The model under review builds one solid part; all positions refer to its coordinate system, in mm. A direction names the side the tool comes from. Give positions to 0.01 mm unless a question says otherwise; leave off trailing zeros. Write each loop counter-clockwise with the first axis right and the second up, starting at its lowest first coordinate (ties: lowest second). Pieces come first, ordered by that corner, then holes. Notation, with made-up numbers: (62, -35) -> (71, -35) arc R16 ccw to (71, -18) -> close; hole circle Ø7 at (56, 57.5). An arc over 180 degrees is marked (long way). Use CSV: the item, a comma, the result in double quotes.
```python
from build123d import *

# Parameters (mm, degrees)
BOSS_EXTRUDE1_DEPTH     = 9.525
SKETCH12_R              = 2.75
CUT_EXTRUDE2_DEPTH      = 278.704385318
CUT_EXTRUDE3_DEPTH      = 291.894698516
CUT_EXTRUDE3_DEPTH_BACK = 291.894698516
SKETCH13_R              = 2.75
SKETCH14_R              = 5
CUT_EXTRUDE4_DEPTH      = 291.894698516


with BuildPart() as part:
    # Sketch1 → Boss-Extrude1 (new, symmetric)
    with BuildSketch(Plane.XY):
        with BuildLine():
            Line((50, 0), (50, 243))
            ThreePointArc((50, 243), (41.213203436, 264.213203436), (20, 273))
            Line((20, 273), (-20, 273))
            ThreePointArc((-20, 273), (-41.213203436, 264.213203436), (-50, 243))
            Line((-50, 243), (-50, 0))
            Line((-50, 0), (-46.825, 0))
            Line((-46.825, 0), (-46.825, 243))
            ThreePointArc((-46.825, 243), (-38.968139405, 261.968139405), (-20, 269.825))
            Line((-20, 269.825), (20, 269.825))
            ThreePointArc((20, 269.825), (38.968139405, 261.968139405), (46.825, 243))
            Line((46.825, 243), (46.825, 0))
            Line((46.825, 0), (50, 0))
        make_face()
    extrude(amount=BOSS_EXTRUDE1_DEPTH, both=True)

    # Sketch12 → Cut-Extrude2 (cut, through all)
    with BuildSketch(Plane(origin=(0, 273, 0), x_dir=(1, 0, 0), z_dir=(0, 1, 0))):
        with Locations(Location((0, 0, 0), (0, 0, 270))):
            Circle(SKETCH12_R)
        with Locations(Location((-15, 0, 0), (0, 0, 270))):
            Circle(SKETCH12_R)
        with Locations(Location((15, 0, 0), (0, 0, 270))):
            Circle(SKETCH12_R)
    extrude(amount=-CUT_EXTRUDE2_DEPTH, mode=Mode.SUBTRACT)

    # Sketch13 → Cut-Extrude3 (cut, two sides: drawn at the far end of the back side and taken through both)
    with BuildSketch(Plane(origin=(50, 0, 0), x_dir=(0, 0, -1), z_dir=(1, 0, 0)).offset(-CUT_EXTRUDE3_DEPTH_BACK)):
        with Locations((0, 220)):
            Circle(SKETCH13_R)
        with Locations((0, 125)):
            Circle(SKETCH13_R)
        with Locations((0, 55)):
            Circle(SKETCH13_R)
    extrude(amount=CUT_EXTRUDE3_DEPTH + CUT_EXTRUDE3_DEPTH_BACK, mode=Mode.SUBTRACT)

    # Sketch14 → Cut-Extrude4 (cut, through all)
    with BuildSketch(Plane(origin=(50, 0, 0), x_dir=(0, 0, -1), z_dir=(1, 0, 0))):
        with Locations((0, 234.175)):
            Circle(SKETCH14_R)
    extrude(amount=-CUT_EXTRUDE4_DEPTH, mode=Mode.SUBTRACT)


solid = part.part
```
Q1. Consider section B-B (x = -15). Write out the cut boundary in (y, z) (3 decimals).
Derived:
outline,"(269.825, -9.525) -> (273, -9.525) -> (273, -2.75) -> (269.825, -2.75) -> close; (269.825, 2.75) -> (273, 2.75) -> (273, 9.525) -> (269.825, 9.525) -> close"
Q2. Insertion check: pin 1 (6.5 mm diameter, centred on x = 15, z = 0, fed in from -Y) (3 decimals); pin 2 (3 mm diameter, centred on x = -28, z = 5.5, fed in from -Y); pin 3 (3 mm diameter, centred on x = 38.5, z = 1, fed in from +Y). Each pin has a flat end and moves straight along its axis. Give the tip position at first contact, or say it passes through.
Derived:
pin 1,"stops at y = 269.825"
pin 2,"stops at y = 268.09"
pin 3,"stops at y = 267.72"
Q3. To check wall thickness, follow probe 1 along X at (y, z) = (226, -4.5) (3 decimals); probe 2 along Z at (x, y) = (47.9, 125) (3 decimals); probe 3 along Y at (x, z) = (47.7, 0) (3 decimals). State the ranges of each line that lie inside material, in increasing order.
Derived:
probe 1,"x = -50 to -46.825, 46.825 to 50"
probe 2,"z = -9.525 to -2.75, 2.75 to 9.525"
probe 3,"y = 0 to 52.25, 57.75 to 122.25, 127.75 to 217.25, 222.75 to 229.175, 239.175 to 254.52"
Q4. Consider section C-C (z = -0.25). State how many separate pieces and enclosed holes the cut face has, then the cut area to 3 significant figures.
Derived:
separate pieces,"12"
enclosed holes,"0"
area,"1,730 mm2"
Q5. Consider section A-A (y = 133.5). Write out the cut boundary in (x, z) (3 decimals).
Derived:
outline,"(-50, -9.525) -> (-46.825, -9.525) -> (-46.825, 9.525) -> (-50, 9.525) -> close; (46.825, -9.525) -> (50, -9.525) -> (50, 9.525) -> (46.825, 9.525) -> close"
Q6. Machinability: for faces 1 (the cylindrical face through (-40.979, 264.445, 0.133)), 2 (the cylindrical face through (-39.176, 261.758, 0.133)), which of the approach directions +Z, -Z, +X, -X, +Y, -Y give a long, thin tool a straight path to every point of the face, cutting with its end or side? Answer none if there is none.
Derived:
face 1,"+Z, -Z, -X, +Y"
face 2,"+Z, -Z, -Y"
Q7. Consider section D-D (x = 30.5). Write out the cut boundary in (y, z) (1 decimal).
Derived:
outline,"(267.7, -9.5) -> (271.1, -9.5) -> (271.1, 9.5) -> (267.7, 9.5) -> close"
Q8. The part is to be moulded in two halves that separate along Z. For faces 3 (the flat face through (48, 137, 9.525)), 4 (the cylindrical face through (-48.435, 217.315, 0.596)), 5 (the cylindrical face through (17.727, 271.435, -0.358)), 6 (the cylindrical face through (41.445, 263.979, 0.133)), say which applies: pulls with the +Z half, pulls with the -Z half, needs draft (parallel to the pull), parting line crosses it, or undercut.
Derived:
face 3,"pulls with the +Z half"
face 4,"undercut"
face 5,"undercut"
face 6,"needs draft"
